```python
from build123d import *

# Parameters (mm, degrees)
SKETCH_1_W      = 40
SKETCH_1_H      = 25.8
EXTRUDE_1_DEPTH = 9.5
SKETCH_2_R      = 1
EXTRUDE_2_DEPTH = 2


with BuildPart() as part:
    # 草图1 → 凸台-拉伸1 (new body)
    with BuildSketch(Plane.XY):
        Rectangle(SKETCH_1_W, SKETCH_1_H)
    extrude(amount=EXTRUDE_1_DEPTH)

    # 草图2 → 凸台-拉伸2 (add)
    with BuildSketch(Plane.XY.offset(9.5)):
        Polygon((-20, 12.9), (20, 12.9), (24.7, 9), (24.7, -9), (20, -12.9), (-20, -12.9), (-24.7, -9), (-24.7, 9), align=None)
        with Locations((-22.6, 9)):
            Circle(SKETCH_2_R, mode=Mode.SUBTRACT)
        with Locations(Location((22.6, 9, 0), (0, 0, 180))):
            Circle(SKETCH_2_R, mode=Mode.SUBTRACT)
        with Locations((22.6, -9)):
            Circle(SKETCH_2_R, mode=Mode.SUBTRACT)
        with Locations(Location((-22.6, -9, 0), (0, 0, 180))):
            Circle(SKETCH_2_R, mode=Mode.SUBTRACT)
    extrude(amount=EXTRUDE_2_DEPTH)


solid = part.part
```
Geometry check sheet. Reference: the model listing, model coordinates, mm. A direction names the side the tool comes from. Give positions to 0.01 mm unless a question says otherwise; leave off trailing zeros. Loops run counter-clockwise (first coordinate to the right, second up) from the corner with the lowest first, then second, coordinate; pieces in that order, holes last. Notation, with made-up numbers: (-32.75, 13) - (-21.75, 13) arc R19 cw to (-21.75, 40) - close; hole circle Ø4 at (-38.75, 26). An arc over 180 degrees is marked (long way). Use CSV: the item, a comma, the result in double quotes. Start each with the question number.
Q1. Release check for a two-part mould opening along X. For faces 1 (the face through (-24.7, 0, 10)), 2 (the face through (-22, 0, 9.5)), 3 (the face through (-21.863, -9.676, 10.486)), 4 (the face through (21.863, -8.324, 10.486)) record: +X half, -X half, draft (parallel to the pull), parting line (faces both ways), or undercut.
Q2. Access from +Z, -Z, +X, -X, +Y, -Y to the whole of each face (thin tool, end or side, straight path). Record for faces 5 (the face through (20, 0, 5)), 6 (the face through (-20, 0, 5)), 7 (the face through (-22.383, 10.923, 10.486)).
Q3. Go/stop test with flat-tipped pins: pin 1 Ø3 at (y, z) = (4, 7) entering from -X; pin 2 Ø1.2 at (x, y) = (22.6, -9) entering from -Z; pin 3 Ø2.5 at (x, y) = (23, -1.5) entering from -Z; pin 4 Ø6 at (y, z) = (-9, 4) entering from +X. Record where each tip stops, or that it passes through.
Q4. Section check B-B, the plane x = -22.6. Record the cut outline in (y, z), and give its area (3 significant figures).
Q5. Section check C-C, the plane z = 7.75. Record the cut outline in (x, y), and give its area (3 significant figures).
Q6. Scan lines: probe 1 along Y at (x, z) = (-22.6, 10.7); probe 2 along Z at (x, y) = (23, -0.75); probe 3 along X at (y, z) = (2.75, 7). Record each from-to range of solid material in increasing order. Write a range as from..to.
Q7. Section check A-A, the plane y = 3. Record the cut outline in (x, z).
Findings below:
1,face 1,"-X half"
1,face 2,"draft"
1,face 3,"undercut"
1,face 4,"undercut"
2,face 5,"-Z, +X, +Y, -Y"
2,face 6,"-Z, -X, +Y, -Y"
2,face 7,"+Z, -Z, -X, +Y"
3,pin 1,"stops at x = -20"
3,pin 2,"passes through"
3,pin 3,"stops at z = 9.5"
3,pin 4,"stops at x = 20"
4,outline,"(-10.74, 9.5) - (-10, 9.5) - (-10, 11.5) - (-10.74, 11.5) - close; (-8, 9.5) - (8, 9.5) - (8, 11.5) - (-8, 11.5) - close; (10, 9.5) - (10.74, 9.5) - (10.74, 11.5) - (10, 11.5) - close"
4,area,"35.0 mm^2"
5,outline,"(-20, -12.9) - (20, -12.9) - (20, 12.9) - (-20, 12.9) - close"
5,area,"1,030 mm^2"
6,probe 1,"y = -10.74..-10, -8..8, 10..10.74"
6,probe 2,"z = 9.5..11.5"
6,probe 3,"x = -20..20"
7,outline,"(-24.7, 9.5) - (-20, 9.5) - (-20, 0) - (20, 0) - (20, 9.5) - (24.7, 9.5) - (24.7, 11.5) - (-24.7, 11.5) - close"
